Part model, mm, in its own coordinate system. A direction names the side the tool comes from. Round coordinates to 2 decimals unless told otherwise and drop trailing zeros. Write each loop counter-clockwise with the first axis right and the second up, starting at its lowest first coordinate (ties: lowest second). Pieces come first, ordered by that corner, then holes. Notation, with made-up numbers: M 1.25,-40 L 60.25,-40 A29 ccw 60.25,-17 Z; hole C -5,-38 d7. An arc over 180 degrees is marked long. Use a Markdown table: item, result. Add a question column.
1) Wall check: probe 1 along Z at (x, y) = (24.5, -31); probe 2 along Y at (x, z) = (31, -0.75); probe 3 along X at (y, z) = (-81.5, 0.4). Give the ranges that are in metal, low to high.
2) Slice it at D-D on y = -5.5. Write the cut outline in (x, z), plus the area to 3 significant figures.
3) Which spindle directions (+Z, -Z, +X, -X, +Y, -Y) get a long thin tool onto all of the face, cutting with end or side? Do faces 1 (the face through (0, 1, 0.25)), 2 (the face through (52.929, -92.604, -0.018)), 3 (the face through (-10, 0.5, 0.4)), 4 (the face through (45.22, -59.3, -9.88)), 5 (the face through (10, 0.5, 0.4)). Say none if no direction does.
4) Slice it at C-C on z = -12. Write the cut outline in (x, y), plus the area to 3 significant figures.
5) Slice it at A-A on y = -81.5. Write the cut outline in (x, z).
6) Two-plate mould, pull along Y, no slides. Class faces 6 (the face through (-13, -1.5, 0)), 7 (the face through (9.62, -44.14, -0.02)), 8 (the face through (29, -68, -18.75)), 9 (the face through (45.35, -84.17, -0.02)): released by +Y, released by -Y, zero draft, split by the parting line, or undercut.
7) Drop flat-ended pins along their axis: P1, Ø0.8, axis at x = -13, z = 0.5, coming from the +Y side; P2, Ø1.5, axis at x = 1.5, y = 0.5, coming from the -Z side; P3, Ø10, axis at y = -57.5, z = -15.5, coming from the -X side; P4, Ø9, axis at x = 46.188, y = -81.5, coming from the +Z side. Give the stop position or say it passes through.
8) Slice it at B-B on x = -9. Write the cut outline in (y, z), plus the area to 3 significant figures.
Autodesk Inventor part; units mm, degrees
ref_plane "YZ Plane" through (0, 0, 0) normal (1, 0, 0) x (0, 1, 0)
ref_plane "XZ Plane" through (0, 0, 0) normal (0, 1, 0) x (-1, 0, 0)
ref_plane "XY Plane" through (0, 0, 0) normal (0, 0, 1) x (1, 0, 0)
sketch "Sketch1" plane through (0, 0, 0) normal (0, 0, 1) x (1, 0, 0)
  line L0 (-16.8629, 0) -> (19.5362, 0)
  line L1 (0, 12.2153) -> (0, -13.8193)
  line L2 (-10, 1.5) -> (10, 1.5)
  line L3 (10, 1.5) -> (10, -1.5)
  line L4 (10, -1.5) -> (-10, -1.5)
  line L5 (-10, -1.5) -> (-10, 1.5)
  point P0 (0, 0)
  point P1 (0, -1.5)
  point P2 (0, 1.5)
  dimension "d0" = 3
  dimension "d1" = 20
sketch "Sketch3" plane through (0, 0, 0) normal (0, 0, 1) x (1, 0, 0)
  line L0 (0, 4.1951) -> (0, -4.771)
  line L1 (15, -1.5) -> (57.438, -75.0048)
  line L2 (-15, -1.5) -> (34.938, -87.9952)
  line L3 (0, -1.5) -> (34.9904, -62.1052)
  arc A0 (34.938, -87.9952) -> (57.438, -75.0048) centre (46.188, -81.5) ccw
  line L4 (-17.5915, 0) -> (22.0991, 0)
  line L5 (-15, -1.5) -> (15, -1.5)
  point P0 (0, -0.2879)
  dimension "d20" = 30
  dimension "d36" = 3
  dimension "d37" = 80
  dimension "d38" = 12.9904
  dimension "d39" = 124.2104
  dimension "d40" = 44.1981
  dimension "d41" = 8.3903
  dimension "d42" = 0.5758
  dimension "d43" = 3
  dimension "d44" = 35.1831
extrude "Extrusion1" add sketch "Sketch3" along normal mid plane 2.5
sketch "Sketch5" plane through (0, 0, 1.25) normal (0, 0, 1) x (1, 0, 0)
  arc A0 (34.938, -87.9952) -> (57.438, -75.0048) centre (46.188, -81.5) ccw
  point P0 (0, 0)
  point P1 (38.391, -42.0144)
hole "Hole1" at (46.188, -81.5, 1.25) direction (0, 0, -1) diameter 5.6 end through all
sketch "Sketch6" plane through (0, 0, 1.25) normal (0, 0, 1) x (1, 0, 0)
  line L0 (21.1799, -20.6847) -> (35.9337, -46.239)
  line L1 (4.4808, -26.761) -> (20.9112, -55.2193)
  line L2 (57.438, -75.0048) -> (15, -1.5)
  line L3 (28.5854, -68.5113) -> (43.7408, -59.7613)
  circle A0 centre (43.7408, -59.7613) radius 1.55
  circle A1 centre (28.5854, -68.5113) radius 1.55
  circle A2 centre (46.188, -81.5) radius 2.8
  line L4 (46.188, -81.5) -> (10.4204, -19.5487)
  line L5 (43.7408, -59.7613) -> (46.188, -81.5)
  point P0 (0, 0)
  point P1 (38.391, -42.0144)
  dimension "d25" = 17.5
  dimension "d26" = 3.1
  dimension "d27" = 3.1
  dimension "d32" = 21.876
extrude "Extrusion3" add sketch "Sketch6" against normal blind 20 contours A1 | A0 L5 L3 | L3 L5 A0
extrude "Extrusion4" add sketch "Sketch1" along normal mid plane 2.5
sketch "Sketch7" plane through (10, -1.5, 1.25) normal (1, 0, 0) x (0, 0, -1)
  line L0 (0, 0) -> (0, 3)
  line L1 (0, 3) -> (2.5, 3)
  line L2 (2.5, 3) -> (2.5, 4)
  line L3 (2.5, 4) -> (0, 4)
  line L4 (0, 4) -> (0, 3)
  line L5 (2.5, 4) -> (3, 3)
  line L6 (3, 3) -> (2.5, 3)
  point P0 (1.25, 1.5)
  dimension "d45" = 1
  dimension "d46" = 0.5
extrude "Extrusion5" add sketch "Sketch7" against normal up to surface (20 mm away)
sketch "Sketch8" plane through (10, -1.5, 1.25) normal (1, 0, 0) x (0, 0, -1)
  line L0 (2.5, 4) -> (0, 4)
  line L1 (1.25, 4) -> (1.25, -0.4591)
  line L2 (1, 4.1974) -> (1.5, 4.1974)
  line L3 (1.5, 4.1974) -> (1.5, 1)
  line L4 (1.5, 1) -> (1, 1)
  line L5 (1, 1) -> (1, 4.1974)
  line L6 (2.5, 0) -> (0, 0)
  point P0 (1.25, 1.5)
  dimension "d49" = 1
  dimension "d50" = 0.5
extrude "Extrusion6" cut sketch "Sketch8" against normal up to surface (20 mm away)
properties part number "bacak"
Entries:
| question | item | result |
|---|---|---|
| 1 | probe 1 | z = -1.25 to 1.25 |
| 1 | probe 2 | y = -81.17 to -29.21 |
| 1 | probe 3 | x = 31.19 to 43.39, 48.99 to 59.18 |
| 2 | outline | M -12.69,-1.25 L 17.31,-1.25 L 17.31,1.25 L -12.69,1.25 Z |
| 2 | area | 75.0 mm^2 |
| 3 | face 1 | +X, -X, +Y |
| 3 | face 2 | +Z, -Z |
| 3 | face 3 | +Z, -Z, -X, +Y |
| 3 | face 4 | -Z |
| 3 | face 5 | +Z, -Z, +X, +Y |
| 4 | outline | C 28.59,-68.51 d3.1; C 43.74,-59.76 d3.1 |
| 4 | area | 15.1 mm^2 |
| 5 | outline | M 31.19,-1.25 L 43.39,-1.25 L 43.39,1.25 L 31.19,1.25 Z; M 48.99,-1.25 L 59.18,-1.25 L 59.18,1.25 L 48.99,1.25 Z |
| 6 | face 6 | released by +Y |
| 6 | face 7 | released by -Y |
| 6 | face 8 | zero draft |
| 6 | face 9 | undercut |
| 7 | P1 | stops at y = -1.5 |
| 7 | P2 | stops at z = -1.25 |
| 7 | P3 | stops at x = 42.19 |
| 7 | P4 | stops at z = 1.25 |
| 8 | outline | M -11.89,-1.25 L 1.5,-1.25 L 1.5,-1.75 L 2.5,-1.25 L 2.5,-0.25 L -0.5,-0.25 L -0.5,0.25 L 2.5,0.25 L 2.5,1.25 L -11.89,1.25 Z |
| 8 | area | 34.7 mm^2 |
